```python
from build123d import *

# Parameters (mm, degrees)
SKETCH1_W           = 300
SKETCH1_H           = 152
BOSS_EXTRUDE1_DEPTH = 61.3
CUT_EXTRUDE1_DEPTH  = 342.850391253
CUT_EXTRUDE2_DEPTH  = 37.06
SHELL2_START        = 2.1
SHELL2_DEPTH        = 59.2
SHELL2_2_DEPTH      = 20.04
BOSS_EXTRUDE3_DEPTH = 59.06
SKETCH10_R          = 2.075
BOSS_EXTRUDE4_DEPTH = 55
SKETCH11_R          = 10.625
BOSS_EXTRUDE7_DEPTH = 41
SKETCH12_W          = 91.45
SKETCH12_H          = 18
BOSS_EXTRUDE8_DEPTH = 60


# Read off the part's stored shape, not the designer's step: Shell2
with BuildPart() as part:
    # Sketch1 → Boss-Extrude1 (new body)
    with BuildSketch(Plane.XY):
        with Locations((150, -76)):
            Rectangle(SKETCH1_W, SKETCH1_H)
    extrude(amount=BOSS_EXTRUDE1_DEPTH)

    # Sketch2 → Cut-Extrude1 (cut, through all)
    with BuildSketch(Plane.XY.offset(61.3)):
        with BuildLine():
            ThreePointArc((106.276631817, -47.688784415), (127.175886892, -13.423863754), (165, 0))
            Line((165, 0), (0, 0))
            Line((0, 0), (0, -152))
            Line((0, -152), (96.53, -152))
            Line((96.53, -152), (84.669267872, -135.896130578))
            ThreePointArc((84.669267872, -135.896130578), (0.080288741, -90.185905943), (89.166858478, -54.015432913))
            ThreePointArc((89.166858478, -54.015432913), (99.658448556, -56.089724813), (106.276631817, -47.688784415))
        make_face()
        with BuildLine():
            Line((209.523701897, -19.780104806), (251.991652277, -30.293700311))
            Line((251.991652277, -30.293700311), (300, -98.856726418))
            Line((300, -98.856726418), (300, 0))
            Line((300, 0), (165, 0))
            ThreePointArc((165, 0), (189.359867491, -5.16755654), (209.523701897, -19.780104806))
        make_face()
        with BuildLine():
            Line((300, -152), (300, -98.856726418))
            Line((300, -98.856726418), (280.413634666, -136.151905638))
            ThreePointArc((280.413634666, -136.151905638), (269.510257097, -147.730229239), (254.19, -152))
            Line((254.19, -152), (300, -152))
        make_face()
    extrude(amount=-CUT_EXTRUDE1_DEPTH, mode=Mode.SUBTRACT)

    # Sketch3 → Cut-Extrude2 (cut)
    with BuildSketch(Plane.XY.offset(61.3)):
        with BuildLine():
            ThreePointArc((105.977880822, -49.211605878), (98.92047416, -56.331219446), (89.166858478, -54.015432913))
            ThreePointArc((89.166858478, -54.015432913), (0.080288741, -90.185905943), (84.669267872, -135.896130578))
            Line((84.669267872, -135.896130578), (96.53, -152))
            Line((96.53, -152), (254.19, -152))
            ThreePointArc((254.19, -152), (269.510257097, -147.730229239), (280.413634666, -136.151905638))
            Line((280.413634666, -136.151905638), (300, -98.856726418))
            Line((300, -98.856726418), (251.991652277, -30.293700311))
            Line((251.991652277, -30.293700311), (209.523701897, -19.780104806))
            ThreePointArc((209.523701897, -19.780104806), (149.343332729, -2.078770991), (106.276631817, -47.688784415))
            ThreePointArc((106.276631817, -47.688784415), (106.15614248, -48.455862107), (105.977880822, -49.211605878))
        make_face()
        with BuildLine():
            ThreePointArc((111.170245832, -48.714719047), (150.648055001, -6.905540075), (205.813393405, -23.131762739))
            Line((205.813393405, -23.131762739), (248.805105887, -33.775023623))
            Line((248.805105887, -33.775023623), (295.06982456, -99.847889378))
            Line((295.06982456, -99.847889378), (275.848412222, -132.766220681))
            ThreePointArc((275.848412222, -132.766220681), (266.986159175, -142.707781738), (254.19, -146.4))
            Line((254.19, -146.4), (98.879937279, -146.4))
            Line((98.879937279, -146.4), (85.901779611, -128.778949784))
            Line((85.901779611, -128.778949784), (81.704299385, -131.870454519))
            ThreePointArc((81.704299385, -131.870454519), (5.072473907, -90.460119595), (85.77880864, -57.692146685))
            ThreePointArc((85.77880864, -57.692146685), (101.106669521, -60.648090535), (111.170245832, -48.714719047))
        make_face(mode=Mode.SUBTRACT)
    extrude(amount=-CUT_EXTRUDE2_DEPTH, mode=Mode.SUBTRACT)

    # Shell2 outline → Shell2 (cut)
    with BuildSketch(Plane.XY.offset(SHELL2_START)):
        with BuildLine():
            Line((99.941363565, -144.3), (254.19, -144.3))
            ThreePointArc((254.19, -144.3), (265.902746491, -140.908301855), (273.990848772, -131.782807449))
            Line((273.990848772, -131.782807449), (292.5780859, -99.950556049))
            Line((292.5780859, -99.950556049), (247.536374557, -35.624325774))
            Line((247.536374557, -35.624325774), (204.678827772, -25.014279675))
            ThreePointArc((204.678827772, -25.014279675), (151.521188692, -8.846000687), (113.233094528, -49.109752168))
            ThreePointArc((113.233094528, -49.109752168), (101.775664547, -62.638918954), (84.37325412, -59.25259838))
            ThreePointArc((84.37325412, -59.25259838), (7.169967657, -90.563406667), (80.458940533, -130.179572699))
            Line((80.458940533, -130.179572699), (86.34730258, -125.842709112))
            Line((86.34730258, -125.842709112), (99.941363565, -144.3))
        make_face()
    extrude(amount=SHELL2_DEPTH, mode=Mode.SUBTRACT)

    # Shell2 2 outline → Shell2 2 (cut)
    with BuildSketch(Plane.XY.offset(SHELL2_START)):
        with BuildLine():
            Line((97.591426286, -149.9), (254.19, -149.9))
            ThreePointArc((254.19, -149.9), (268.424080868, -145.932947626), (278.554430318, -135.175504495))
            Line((278.554430318, -135.175504495), (297.545882937, -99.013122297))
            Line((297.545882937, -99.013122297), (250.722920948, -32.143002462))
            Line((250.722920948, -32.143002462), (208.389700931, -21.662761535))
            ThreePointArc((208.389700931, -21.662761535), (150.241547582, -4.012518522), (108.350090196, -48.033475058))
            ThreePointArc((108.350090196, -48.033475058), (100.340566871, -58.076361401), (87.743795173, -55.559742089))
            ThreePointArc((87.743795173, -55.559742089), (2.130315246, -91.350316403), (85.089165222, -132.925096807))
            Line((85.089165222, -132.925096807), (97.591426286, -149.9))
        make_face()
        with BuildLine():
            ThreePointArc((273.990848772, -131.782807449), (265.902746491, -140.908301855), (254.19, -144.3))
            Line((254.19, -144.3), (99.941363565, -144.3))
            Line((99.941363565, -144.3), (86.34730258, -125.842709112))
            Line((86.34730258, -125.842709112), (80.458940533, -130.179572699))
            ThreePointArc((80.458940533, -130.179572699), (7.169967657, -90.563406667), (84.37325412, -59.25259838))
            ThreePointArc((84.37325412, -59.25259838), (101.775664547, -62.638918954), (113.233094528, -49.109752168))
            ThreePointArc((113.233094528, -49.109752168), (151.521188692, -8.846000687), (204.678827772, -25.014279675))
            Line((204.678827772, -25.014279675), (247.536374557, -35.624325774))
            Line((247.536374557, -35.624325774), (292.5780859, -99.950556049))
            Line((292.5780859, -99.950556049), (273.990848772, -131.782807449))
        make_face(mode=Mode.SUBTRACT)
    extrude(amount=SHELL2_2_DEPTH, mode=Mode.SUBTRACT)

    # Sketch9 → Boss-Extrude3 (add)
    with BuildSketch(Plane.XY.offset(61.3)):
        Polygon((247.536374557, -35.624325774), (219.726374557, -35.624325774), (264.7680859, -99.950556049), (292.5780859, -99.950556049), (248.135467364, -36.479918971), align=None)
    extrude(amount=-BOSS_EXTRUDE3_DEPTH)

    # Sketch10 → Boss-Extrude4 (add)
    with BuildSketch(Plane.XY.offset(2.1)):
        with Locations((118, -47.741938271)):
            Circle(SKETCH10_R)
        with Locations((207.29, -47.741938271)):
            Circle(SKETCH10_R)
        with Locations((162.650383795, -12.633773594)):
            Circle(SKETCH10_R)
    extrude(amount=BOSS_EXTRUDE4_DEPTH)

    # Sketch11 → Boss-Extrude7 (add)
    with BuildSketch(Plane.XY.offset(2.1)):
        with Locations((104.050993742, -74.01432733)):
            Circle(SKETCH11_R)
    extrude(amount=BOSS_EXTRUDE7_DEPTH)

    # Sketch12 → Boss-Extrude8 (add)
    with BuildSketch(Plane.XY.offset(2.1)):
        with Locations((170.666363565, -135.3)):
            Rectangle(SKETCH12_W, SKETCH12_H)
        with BuildLine():
            Line((106.891363565, -144.3), (121.411363565, -144.3))
            ThreePointArc((121.411363565, -144.3), (114.151363565, -131.75824963), (106.891363565, -144.3))
        make_face()
        with BuildLine():
            Line((219.350413724, -144.3), (233.870413724, -144.3))
            ThreePointArc((233.870413724, -144.3), (226.610413724, -131.046495008), (219.350413724, -144.3))
        make_face()
    extrude(amount=BOSS_EXTRUDE8_DEPTH)


solid = part.part
```
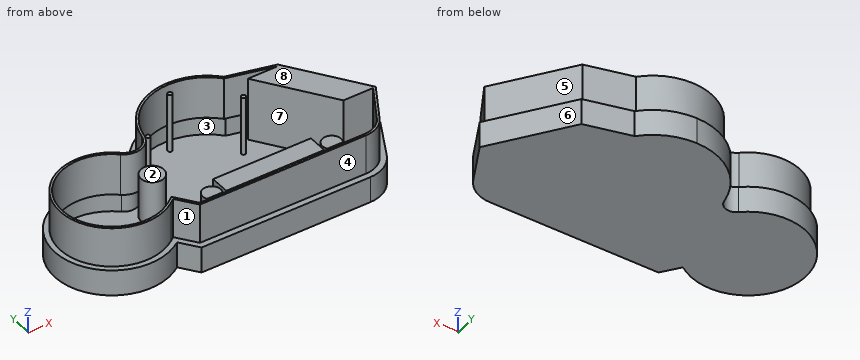
Here's how the part is built. I have some questions about the finished solid (model axes, mm). Face numbers are marked on the shaded views. A direction names the side the tool comes from. Give positions to 0.01 mm unless a question says otherwise; leave off trailing zeros. Loops run counter-clockwise (first coordinate to the right, second up) from the corner with the lowest first, then second, coordinate; pieces in that order, holes last. Notation, with made-up numbers: M 3.25,-12 L 27.25,-12 A16 cw 27.25,9 Z; hole C -18.5,-4 d9. An arc over 180 degrees is marked long. Return JSON: item names as keys, results as strings.
Item 1: On a 3-axis mill with a long thin cutter (end or side, diameter ignored), from which of +Z, -Z, +X, -X, +Y, -Y can I reach the whole of each face in a straight line? I mean the marked faces 1, 2, 3, 4 and 5. Say none if no direction works.
A:
{"face 1": "+Z, -Y", "face 2": "+Z", "face 3": "none", "face 4": "+Z, +X, -X, -Y", "face 5": "+Z, +X, +Y"}
Item 2: Imagine slicing it at A-A on z = 31. State how many separate pieces and enclosed holes the cut face has, then the cut area to 3 significant figures.
A:
{"separate pieces": "5", "enclosed holes": "1", "area": "5,750 mm^2"}
Item 3: I'm going to push flat-ended pins straight in: pin 1 Ø23.5 at (x, y) = (100, -72) entering from +Z; pin 2 Ø5.5 at (y, z) = (-136.5, 21) entering from +X; pin 3 Ø12 at (y, z) = (-30.5, 25.5) entering from -X. Where does each tip first touch, or does it pass through?
A:
{"pin 1": "stops at z = 61.3", "pin 2": "stops at x = 281.68", "pin 3": "stops at x = 109.85"}
Item 4: Imagine slicing it at C-C on x = 53.15. List the corners of the cut face in (y, z) for me, then the cut area to 3 significant figures.
A:
{"outline": "M -146.25,0 L -39.95,0 L -39.95,24.24 L -44.95,24.24 L -44.95,61.3 L -47.05,61.3 L -47.05,22.14 L -42.05,22.14 L -42.05,2.1 L -144.15,2.1 L -144.15,22.14 L -139.15,22.14 L -139.15,61.3 L -141.25,61.3 L -141.25,24.24 L -146.25,24.24 Z", "area": "493 mm^2"}
Item 5: Please list where these lines run through material, in increasing order: line 1 (Y direction, x = 205.5, z = 40); line 2 (Z direction, x = 278.5, y = -126.5); line 3 (X direction, y = -57.5, z = 19.5).
A:
{"line 1": "y = -146.4 to -126.3, -48.79 to -46.69, -25.22 to -22.79", "line 2": "z = 0 to 2.1, 22.14 to 61.3", "line 3": "x = 13.69 to 16.56, 90.54 to 101.67, 235.04 to 262.85, 268.48 to 271.04"}
Item 6: Thinking about a two-plate mould opening in X: for the marked faces 6, 7 and 8, which applies, released by +X, released by -X, zero draft, split by the parting line, or undercut?
A:
{"face 6": "released by +X", "face 7": "undercut", "face 8": "zero draft"}
Item 7: Imagine slicing it at B-B on x = 225. List the corners of the cut face in (y, z) for me, then the cut area to 3 significant figures.
A:
{"outline": "M -152,0 L -23.61,0 L -23.61,24.24 L -27.88,24.24 L -27.88,61.3 L -30.05,61.3 L -30.05,22.14 L -25.77,22.14 L -25.77,2.1 L -131.2,2.1 L -131.2,62.1 L -144.3,62.1 L -144.3,61.3 L -146.4,61.3 L -146.4,24.24 L -152,24.24 Z; M -43.16,2.24 L -35.62,2.24 L -35.62,61.3 L -43.16,61.3 Z; hole M -149.9,2.1 L -144.3,2.1 L -144.3,22.14 L -149.9,22.14 Z", "area": "1,770 mm^2"}
